Read the model definition and answer for the solid it produces. Units are mm, in the model's axes. A direction names the side the tool comes from. Coordinates: 2 decimals unless noted, no trailing zeros. Loops run counter-clockwise (first coordinate to the right, second up) from the corner with the lowest first, then second, coordinate; pieces in that order, holes last.
Autodesk Inventor part; units mm, degrees
ref_plane "YZ Plane" through (0, 0, 0) normal (1, 0, 0) x (0, 1, 0)
ref_plane "XZ Plane" through (0, 0, 0) normal (0, 1, 0) x (-1, 0, 0)
ref_plane "XY Plane" through (0, 0, 0) normal (0, 0, 1) x (1, 0, 0)
sketch "Sketch1" plane through (0, 0, 0) normal (0, 0, 1) x (1, 0, 0)
  line L0 (-42.5, 37.5) -> (42.5, 37.5)
  line L1 (42.5, 37.5) -> (42.5, -37.5)
  line L2 (42.5, -37.5) -> (-42.5, -37.5)
  line L3 (-42.5, -37.5) -> (-42.5, 37.5)
  point P0 (0, 0)
  dimension "d0" = 85
  dimension "d1" = 75
  dimension "d2" = 37.5
  dimension "d3" = 42.5
extrude "Extrusion1" add sketch "Sketch1" along normal blind 7.5
sketch "Sketch2" plane through (0, 0, 7.5) normal (0, 0, 1) x (1, 0, 0)
  point P0 (0, 0)
  point P1 (20, -33.75)
  point P2 (-20, -33.75)
  point P3 (-20, 33.75)
  point P4 (20, 33.75)
  dimension "d6" = 40
  dimension "d7" = 20
  dimension "d8" = 67.5
  dimension "d9" = 33.75
hole "Hole1" at (20, -33.75, 7.5) at (-20, -33.75, 7.5) at (-20, 33.75, 7.5) at (20, 33.75, 7.5) direction (0, 0, -1) diameter 4.5 depth 9.525 tip angle 118
sketch "Sketch3" plane through (0, 0, 7.5) normal (0, 0, 1) x (1, 0, 0)
  line L0 (-37.5, -30) -> (37.5, -30)
  line L1 (37.5, -30) -> (37.5, 30)
  line L2 (37.5, 30) -> (-37.5, 30)
  line L3 (-37.5, 30) -> (-37.5, -30)
  line L4 (-32.5, -25) -> (32.5, -25)
  line L5 (32.5, -25) -> (32.5, 25)
  line L6 (32.5, 25) -> (-32.5, 25)
  line L7 (-32.5, 25) -> (-32.5, -25)
  point P0 (0, 0)
  dimension "d19" = 75
  dimension "d22" = 60
  dimension "d23" = 30
  dimension "d24" = 5
  dimension "d26" = 37.5
  dimension "d27" = 5
  dimension "d29" = 5
  dimension "d30" = 5
extrude "Extrusion2" cut sketch "Sketch3" against normal blind 6
equation "\"d27\" = d24"
equation "\"d29\" = d24"
equation "\"d30\" = d24"
properties part number "smallSampleHolder"
Item 1: A cutting plane is placed at A-A on x = -20. Determine the outline of the cut face in (y, z), then the cut area to 3 significant figures.
Numbers:
outline: (-37.5, 0) - (-36, 0) - (-36, 7.5) - (-37.5, 7.5) - close; (-31.5, 0) - (31.5, 0) - (31.5, 7.5) - (30, 7.5) - (30, 1.5) - (25, 1.5) - (25, 7.5) - (-25, 7.5) - (-25, 1.5) - (-30, 1.5) - (-30, 7.5) - (-31.5, 7.5) - close; (36, 0) - (37.5, 0) - (37.5, 7.5) - (36, 7.5) - close
area: 435 mm2
Item 2: A cutting plane is placed at C-C on x = -2. Determine the outline of the cut face in (y, z), then the cut area to 4 significant figures.
Numbers:
outline: (-37.5, 0) - (37.5, 0) - (37.5, 7.5) - (30, 7.5) - (30, 1.5) - (25, 1.5) - (25, 7.5) - (-25, 7.5) - (-25, 1.5) - (-30, 1.5) - (-30, 7.5) - (-37.5, 7.5) - close
area: 502.5 mm2
Item 3: Which of the six approach directions +Z, -Z, +X, -X, +Y, -Y give full straight-line access (tool end or side, diameter ignored) to faces 1 (the face through (21.996, -34.788, 3.698)), 2 (the face through (37.5, 0, 5))?
Numbers:
face 1: +Z, -Z
face 2: +Z
Item 4: Given pin 1 (6 mm diameter, centred on x = 20, y = -33.75, fed in from -Z), flat-ended and moving along its own axis, determine where the tip first touches the part or whether it passes through.
Numbers:
pin 1: stops at z = 0
Item 5: Determine the mould class of faces 3 (the face through (0, 0, 7.5)), 4 (the face through (1, 30, 5)), 5 (the face through (0, -25, 5)), 6 (the face through (-42.5, -1, 4)) for opening direction X: released by +X, released by -X, zero draft, split by the parting line, or undercut.
Numbers:
face 3: zero draft
face 4: undercut
face 5: undercut
face 6: released by -X
Item 6: A cutting plane is placed at B-B on y = -33.75. Determine the outline of the cut face in (x, z), then the cut area to 3 significant figures.
Numbers:
outline: (-42.5, 0) - (-22.25, 0) - (-22.25, 7.5) - (-42.5, 7.5) - close; (-17.75, 0) - (17.75, 0) - (17.75, 7.5) - (-17.75, 7.5) - close; (22.25, 0) - (42.5, 0) - (42.5, 7.5) - (22.25, 7.5) - close
area: 570 mm2
Item 7: Find the intervals of material crossed by line 1 along Y through (x, z) = (24, 3); line 2 along Y through (x, z) = (20, 2); line 3 along X through (y, z) = (17, 5), in increasing order.
Numbers:
line 1: y = -37.5 to -30, -25 to 25, 30 to 37.5
line 2: y = -37.5 to -36, -31.5 to -30, -25 to 25, 30 to 31.5, 36 to 37.5
line 3: x = -42.5 to -37.5, -32.5 to 32.5, 37.5 to 42.5
Item 8: A cutting plane is placed at D-D on y = -15.5. Determine the outline of the cut face in (x, z).
Numbers:
outline: (-42.5, 0) - (42.5, 0) - (42.5, 7.5) - (37.5, 7.5) - (37.5, 1.5) - (32.5, 1.5) - (32.5, 7.5) - (-32.5, 7.5) - (-32.5, 1.5) - (-37.5, 1.5) - (-37.5, 7.5) - (-42.5, 7.5) - close
